Check sheet for the modelled part. Datum: model origin and axes. Units: mm. Round coordinates to 2 decimals unless told otherwise and drop trailing zeros. Order: outer loops, then holes, each group sorted by start corner. A loop starts at its lowest first (then second) coordinate and runs counter-clockwise, first axis right, second up.
(1) Thickness scan on probe 1 along Z at (x, y) = (-15, -14.5); probe 2 along Z at (x, y) = (-22.5, -13.5); probe 3 along X at (y, z) = (-13.5, -16.5). Record the ranges inside material, lowest first.
(2) Sectioned sample at B-B, the plane y = -9.25. Enter the section's corners in (x, z).
(3) Sectioned sample at A-A, the plane z = -49. Enter the section's corners in (x, y).
(4) Depth check by flat-ended pin: pin 1 (5 mm diameter, centred on y = -3.5, z = -25, fed in from +X). Enter the tip coordinate at first touch or a pass-through.
(5) Sectioned sample at D-D, the plane z = 26.5. Enter the section's corners in (x, y).
(6) Sectioned sample at C-C, the plane x = -109. Enter the section's corners in (y, z).
```python
from build123d import *

# Parameters (mm, degrees)
F1_DEPTH = 19.05


with BuildPart() as f1:
    # F0 (on Front) → F1 (new body)
    with BuildSketch(Plane.XZ):
        with BuildLine():
            Line((328.634582, 63.5), (-56.863403, 63.5))
            Line((-56.863403, 63.5), (-332.736589, -13.935924))
            ThreePointArc((-332.736589, -13.935924), (-350.018995, -41.943488), (-325.150903, -63.5))
            Line((-325.150903, -63.5), (-157.95625, -63.5))
            ThreePointArc((-157.95625, -63.5), (-5.55625, -31.82137), (146.84375, -63.5))
            Line((146.84375, -63.5), (328.634582, -63.5))
            ThreePointArc((328.634582, -63.5), (335.963356, -61.172033), (340.605336, -55.041584))
            ThreePointArc((340.605336, -55.041584), (350.068505, 0), (340.605336, 55.041584))
            ThreePointArc((340.605336, 55.041584), (335.963356, 61.172033), (328.634582, 63.5))
        make_face()
    extrude(amount=F1_DEPTH)


solid = f1.part
```
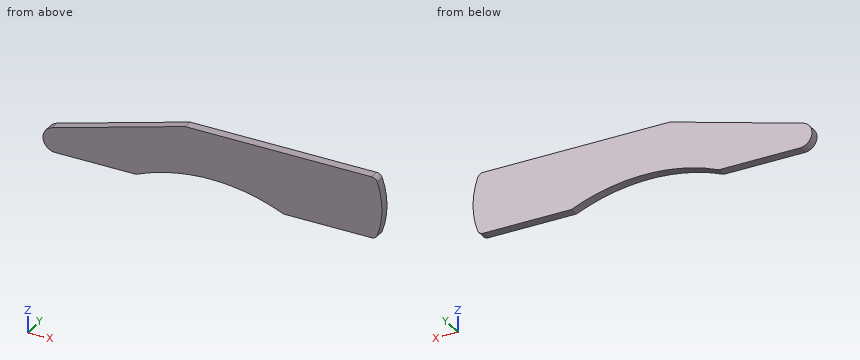
Derived:
1. probe 1: z = -31.94 to 63.5
1. probe 2: z = -32.2 to 63.5
1. probe 3: x = -338.27 to 349.24
2. outline: (-332.74, -13.94) arc R25.4 ccw to (-325.15, -63.5) - (-157.96, -63.5) arc R382.42 cw to (146.84, -63.5) - (328.63, -63.5) arc R12.7 ccw to (340.61, -55.04) arc R164.8 ccw to (340.61, 55.04) arc R12.7 ccw to (328.63, 63.5) - (-56.86, 63.5) - close
3. outline: (-347.85, -19.05) - (-118.89, -19.05) - (-118.89, 0) - (-347.85, 0) - close; (107.77, -19.05) - (342.62, -19.05) - (342.62, 0) - (107.77, 0) - close
4. pin 1: stops at x = 348.53
5. outline: (-188.68, -19.05) - (347.92, -19.05) - (347.92, 0) - (-188.68, 0) - close
6. outline: (-19.05, -46.08) - (0, -46.08) - (0, 48.87) - (-19.05, 48.87) - close
